```python
from build123d import *

# Parameters (mm, degrees)
SKETCH2_R           = 15
BOSS_EXTRUDE1_DEPTH = 10
CUT_EXTRUDE1_START  = -7
SKETCH3_R           = 15
SKETCH3_R_2         = 12.5
CUT_EXTRUDE1_DEPTH  = 7
SKETCH4_R           = 7.5
BOSS_EXTRUDE4_DEPTH = 17.695


with BuildPart() as part:
    # Sketch2 → Boss-Extrude1 (new body)
    with BuildSketch(Plane.XY):
        Circle(SKETCH2_R)
    extrude(amount=BOSS_EXTRUDE1_DEPTH)

    # Sketch3 → Cut-Extrude1 (cut)
    with BuildSketch(Plane.XY.offset(10).offset(CUT_EXTRUDE1_START)):
        Circle(SKETCH3_R)
        Circle(SKETCH3_R_2, mode=Mode.SUBTRACT)
    extrude(amount=CUT_EXTRUDE1_DEPTH, mode=Mode.SUBTRACT)

    # Sketch4 → Boss-Extrude4 (add)
    with BuildSketch(Plane.XY.offset(10)):
        Circle(SKETCH4_R)
    extrude(amount=BOSS_EXTRUDE4_DEPTH)


solid = part.part
```
The listing builds one solid part. Answer for the finished solid, in the listing's coordinates (mm). A direction names the side the tool comes from. Give positions to 0.01 mm unless a question says otherwise; leave off trailing zeros. Order: outer loops, then holes, each group sorted by start corner. A loop starts at its lowest first (then second) coordinate and runs counter-clockwise, first axis right, second up.
Item 1: The part is cut by section C-C, the plane z = 5.25. Give the vertices of the cut face in (x, y), and give its area (3 significant figures).
From the geometry:
outline: circle Ø25 at (0, 0)
area: 491 mm2
Item 2: Given pin 1 Ø1.5 at (x, y) = (8, -5) entering from +Z; pin 2 Ø8 at (x, z) = (10.5, 22) entering from +Y; pin 3 Ø3 at (y, z) = (-5.5, 7.5) entering from -X, each flat-ended and moving along its own axis, determine where each tip first touches the part or whether it passes through.
From the geometry:
pin 1: stops at z = 10
pin 2: stops at y = 3.74
pin 3: stops at x = -11.84
Item 3: Find the intervals of material crossed by probe 1 along Z at (x, y) = (-7.25, -4.25); probe 2 along Z at (x, y) = (-12.5, 2.75); probe 3 along X at (y, z) = (-6.5, 5), in increasing order.
From the geometry:
probe 1: z = 0 to 10
probe 2: z = 0 to 3
probe 3: x = -10.68 to 10.68
Item 4: The part is cut by section D-D, the plane x = -11.5. Give the vertices of the cut face in (y, z).
From the geometry:
outline: (-9.63, 0) - (9.63, 0) - (9.63, 3) - (4.9, 3) - (4.9, 10) - (-4.9, 10) - (-4.9, 3) - (-9.63, 3) - close
Item 5: The part is cut by section A-A, the plane y = 0. Give the vertices of the cut face in (x, z) (3 decimals), and give its area (3 significant figures).
From the geometry:
outline: (-15, 0) - (15, 0) - (15, 3) - (12.5, 3) - (12.5, 10) - (7.5, 10) - (7.5, 27.695) - (-7.5, 27.695) - (-7.5, 10) - (-12.5, 10) - (-12.5, 3) - (-15, 3) - close
area: 530 mm2
Item 6: Which of the six approach directions +Z, -Z, +X, -X, +Y, -Y give full straight-line access (tool end or side, diameter ignored) to faces 1 (the face through (0, 0, 27.695)), 2 (the face through (-7.493, 0.33, 18.724))?
From the geometry:
face 1: +Z, +X, -X, +Y, -Y
face 2: +Z
